Build history of the part. All positions in model axes, mm. Face numbers are marked on the shaded views. A direction names the side the tool comes from. Round coordinates to 2 decimals unless told otherwise and drop trailing zeros. Write each loop counter-clockwise with the first axis right and the second up, starting at its lowest first coordinate (ties: lowest second). Pieces come first, ordered by that corner, then holes. Notation, with made-up numbers: M 68,24 L 101,24 A7 cw 101,34 Z; hole C -38.75,23 d11. An arc over 180 degrees is marked long. Write item = value, one per line. Start each with the question number.
Q1. Band-saw the part on A-A on x = 5.75. Write the cut outline in (y, z), plus the area to 3 significant figures.
Q2. Drop flat-ended pins along their axis: P1, Ø8, axis at x = 5.5, z = -12.5, coming from the -Y side; P2, Ø10, axis at x = 13, z = -14.5, coming from the -Y side; P3, Ø3, axis at x = 16.5, z = -2.5, coming from the -Y side; P4, Ø10, axis at x = 9, y = 9, coming from the -Z side. Give the stop position or say it passes through.
Q3. Pull direction Y, two halves, no side cores. Call the marked faces 1, 2, 3 and 4: released by +Y, released by -Y, zero draft, split by the parting line, or undercut.
Q4. Band-saw the part on C-C on z = 26. Write the cut outline in (x, y).
Q5. Band-saw the part on B-B on y = -8.75. Write the cut outline in (x, z), plus the area to 3 significant figures.
Q6. Tool access for the marked faces 5, 6 and 7: list every direction of +Z, -Z, +X, -X, +Y, -Y with a clear straight run to the whole face (end or side of a thin tool).
Q7. Probe L1, parallel to Y at x = 4.75, z = -30; L2, parallel to Z at x = 12.75, y = -1.75; L3, parallel to Z at x = 3, y = -1.5. List the from-to ranges inside material, lowest first.
Q8. Band-saw the part on D-D on y = 10. Write the cut outline in (x, z).
```python
from build123d import *

# Parameters (mm, degrees)
SKETCH1_R           = 7.5
BOSS_EXTRUDE1_DEPTH = 20
SKETCH2_W           = 10
SKETCH2_H           = 40
CUT_EXTRUDE1_DEPTH  = 53.239831546


with BuildPart() as part:
    # Sketch1 → Boss-Extrude1 (new body)
    with BuildSketch(Plane(origin=(0, 0, 0), x_dir=(0, 0, -1), z_dir=(1, 0, 0))):
        with BuildLine():
            Line((-19, -13.5), (-12, -1.5))
            Line((-12, -1.5), (12, -1.5))
            Line((12, -1.5), (19, -13.5))
            Line((19, -13.5), (40, -13.5))
            Line((40, -13.5), (40, 3.5))
            ThreePointArc((40, 3.5), (37.071067812, 10.571067812), (30, 13.5))
            Line((30, 13.5), (-30, 13.5))
            ThreePointArc((-30, 13.5), (-37.071067812, 10.571067812), (-40, 3.5))
            Line((-40, 3.5), (-40, -13.5))
            Line((-40, -13.5), (-19, -13.5))
        make_face()
        with Locations((-30, 3.5)):
            Circle(SKETCH1_R, mode=Mode.SUBTRACT)
        with Locations((30, 3.5)):
            Circle(SKETCH1_R, mode=Mode.SUBTRACT)
    extrude(amount=BOSS_EXTRUDE1_DEPTH)

    # Sketch2 → Cut-Extrude1 (cut, through all)
    with BuildSketch(Plane(origin=(0, 13.5, 0), x_dir=(1, 0, 0), z_dir=(0, 1, 0))):
        with Locations((5, 0)):
            Rectangle(SKETCH2_W, SKETCH2_H)
    extrude(amount=-CUT_EXTRUDE1_DEPTH, mode=Mode.SUBTRACT)


solid = part.part
```
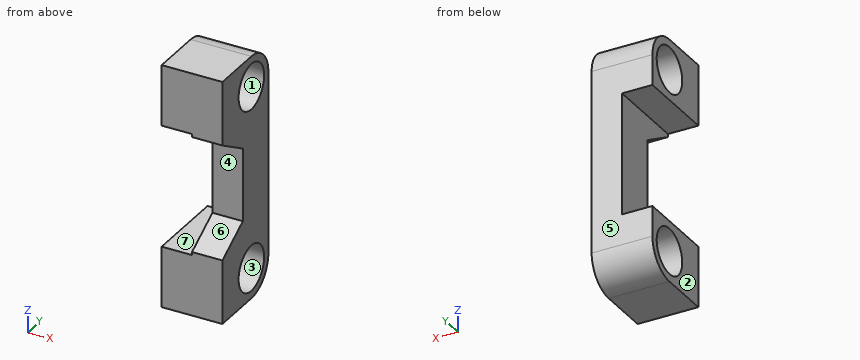
Conclusion:
q1.outline = M -13.5,-40 L 3.5,-40 A10 ccw 13.5,-30 L 13.5,-20 L -13.5,-20 Z; M -13.5,20 L 13.5,20 L 13.5,30 A10 ccw 3.5,40 L -13.5,40 Z; hole C 3.5,-30 d15; hole C 3.5,30 d15
q1.area = 684 mm^2
q2.P1 = through
q2.P2 = -13.5
q2.P3 = -1.5
q2.P4 = -39.99
q3.face_1 = undercut
q3.face_2 = zero draft
q3.face_3 = undercut
q3.face_4 = released by -Y
q4.outline = M 0,-13.5 L 20,-13.5 L 20,-2.84 L 0,-2.84 Z; M 0,9.84 L 20,9.84 L 20,13.5 L 0,13.5 Z
q5.outline = M 0,-40 L 20,-40 L 20,-16.23 L 10,-16.23 L 10,-20 L 0,-20 Z; M 0,20 L 10,20 L 10,16.23 L 20,16.23 L 20,40 L 0,40 Z
q5.area = 875 mm^2
q6.face_5 = +Z, -Z, +X, -X, +Y
q6.face_6 = +X, -X, -Y
q6.face_7 = -X, +Y, -Y
q7.L1 = -13.5 to -4, 11 to 13.5
q7.L2 = -40 to -35.36, -24.64 to -12.15, 12.15 to 24.64, 35.36 to 40
q7.L3 = -40 to -35.59, -24.41 to -20, 20 to 24.41, 35.59 to 40
q8.outline = M 0,-37.6 L 20,-37.6 L 20,-33.74 L 0,-33.74 Z; M 0,-26.26 L 20,-26.26 L 20,26.26 L 0,26.26 L 0,20 L 10,20 L 10,-20 L 0,-20 Z; M 0,33.74 L 20,33.74 L 20,37.6 L 0,37.6 Z
